```python
from build123d import *

# Parameters (mm, degrees)
SKETCH1_W            = 50.8
SKETCH1_H            = 88.9
BOSS_EXTRUDE1_DEPTH  = 19.05
CUT_EXTRUDE1_DEPTH   = 12.7
LPATTERN1_COUNT      = 3
LPATTERN1_PITCH      = 50.8
LPATTERN1_COUNT_DIR2 = 2
LPATTERN1_PITCH_DIR2 = 88.9


with BuildPart() as part:
    # Sketch1 → Boss-Extrude1 (new body)
    with BuildSketch(Plane.XY):
        Rectangle(SKETCH1_W, SKETCH1_H)
    boss_extrude1 = extrude(amount=BOSS_EXTRUDE1_DEPTH)

    # Sketch2 → Cut-Extrude1 (cut)
    with BuildSketch(Plane.XY.offset(19.05)):
        with BuildLine():
            ThreePointArc((-17.960512242, -12.7), (0, -38.1), (17.960512242, -12.7))
            ThreePointArc((17.960512242, -12.7), (6.717373, 11.89995), (0, 38.1))
            ThreePointArc((0, 38.1), (-6.717373, 11.89995), (-17.960512242, -12.7))
        make_face()
    cut_extrude1 = extrude(amount=-CUT_EXTRUDE1_DEPTH, mode=Mode.SUBTRACT)

    # LPattern1: Boss-Extrude1, Cut-Extrude1 3 × 2
    with Locations(*[(i * LPATTERN1_PITCH, j * LPATTERN1_PITCH_DIR2, 0) for i in range(LPATTERN1_COUNT) for j in range(LPATTERN1_COUNT_DIR2) if (i, j) != (0, 0)]):
        add(boss_extrude1)
        add(cut_extrude1, mode=Mode.SUBTRACT)


solid = part.part
```
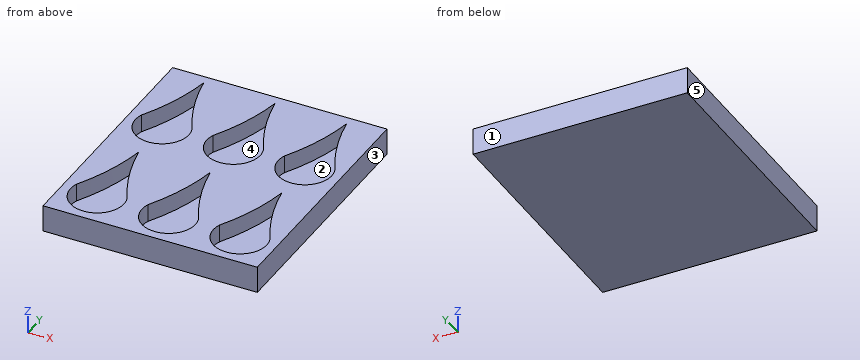
CAD build for the part. Positions are in the model's coordinates, mm. Face numbers are marked on the shaded views. A direction names the side the tool comes from. Round coordinates to 2 decimals unless told otherwise and drop trailing zeros. Order: outer loops, then holes, each group sorted by start corner. A loop starts at its lowest first (then second) coordinate and runs counter-clockwise, first axis right, second up. Notation, with made-up numbers: (-0.5, -0.75) - (25.5, -0.75) arc R17 cw to (25.5, 8.25) - close; hole circle Ø10 at (86, 36). An arc over 180 degrees is marked (long way). Answer as CSV lines item,"result". Start each with the question number.
1. Tool access for the marked faces 4 and 5: list every direction of +Z, -Z, +X, -X, +Y, -Y with a clear straight run to the whole face (end or side of a thin tool).
2. Drill centre lines: L1, parallel to X at y = -19.05, z = 13.75; L2, parallel to X at y = 31.5, z = 10.25; L3, parallel to Y at x = 42, z = 8.5. Where is each one in solid material? Low to high. Write a range as [from, to].
3. Saw through at D-D, the plane y = 110. Write the cut outline in (x, z), and give its area (3 significant figures).
4. Pull direction Y, two halves, no side cores. Call the marked faces 1, 2 and 3: +Y half, -Y half, draft (parallel to the pull), parting line (faces both ways), or undercut.
5. Saw through at B-B, the plane y = -19.05. Write the cut outline in (x, z), and give its area (3 significant figures).
6. Saw through at C-C, the plane x = 113. Write the cut outline in (y, z), and give its area (3 significant figures).
7. Saw through at A-A, the plane z = 16. Write the cut outline in (x, y).
Model answer:
1,face 4,"+Z"
1,face 5,"+Z, -Z, -X, +Y, -Y"
2,L1,"x = [-25.4, -19.05], [19.05, 31.75], [69.85, 82.55], [120.65, 127]"
2,L2,"x = [-25.4, -1.23], [1.23, 49.57], [52.03, 100.37], [102.83, 127]"
2,L3,"y = [-44.45, -35.95], [6.35, 52.95], [95.25, 133.35]"
3,outline,"(-25.4, 0) - (127, 0) - (127, 19.05) - (105.39, 19.05) - (105.39, 6.35) - (97.81, 6.35) - (97.81, 19.05) - (54.59, 19.05) - (54.59, 6.35) - (47.01, 6.35) - (47.01, 19.05) - (3.79, 19.05) - (3.79, 6.35) - (-3.79, 6.35) - (-3.79, 19.05) - (-25.4, 19.05) - close"
3,area,"2,610 mm²"
4,face 1,"+Y half"
4,face 2,"undercut"
4,face 3,"draft"
5,outline,"(-25.4, 0) - (127, 0) - (127, 19.05) - (120.65, 19.05) - (120.65, 6.35) - (82.55, 6.35) - (82.55, 19.05) - (69.85, 19.05) - (69.85, 6.35) - (31.75, 6.35) - (31.75, 19.05) - (19.05, 19.05) - (19.05, 6.35) - (-19.05, 6.35) - (-19.05, 19.05) - (-25.4, 19.05) - close"
5,area,"1,450 mm²"
6,outline,"(-44.45, 0) - (133.35, 0) - (133.35, 19.05) - (89.12, 19.05) - (89.12, 6.35) - (54.59, 6.35) - (54.59, 19.05) - (0.22, 19.05) - (0.22, 6.35) - (-34.31, 6.35) - (-34.31, 19.05) - (-44.45, 19.05) - close"
6,area,"2,510 mm²"
7,outline,"(-25.4, -44.45) - (127, -44.45) - (127, 133.35) - (-25.4, 133.35) - close; hole (-17.96, -12.7) arc R19.05 ccw (long way) to (17.96, -12.7) arc R152.4 cw to (0, 38.1) arc R152.4 cw to start; hole (-17.96, 76.2) arc R19.05 ccw (long way) to (17.96, 76.2) arc R152.4 cw to (0, 127) arc R152.4 cw to start; hole (32.84, -12.7) arc R19.05 ccw (long way) to (68.76, -12.7) arc R152.4 cw to (50.8, 38.1) arc R152.4 cw to start; hole (32.84, 76.2) arc R19.05 ccw (long way) to (68.76, 76.2) arc R152.4 cw to (50.8, 127) arc R152.4 cw to start; hole (83.64, -12.7) arc R19.05 ccw (long way) to (119.56, -12.7) arc R152.4 cw to (101.6, 38.1) arc R152.4 cw to start; hole (83.64, 76.2) arc R19.05 ccw (long way) to (119.56, 76.2) arc R152.4 cw to (101.6, 127) arc R152.4 cw to start"
